Here's the drawing with two shaded views (mm, measured from the low corner). I have some questions. A direction names the side the tool comes from. Give positions to 0.01 mm unless a question says otherwise; leave off trailing zeros. Write each loop counter-clockwise with the first axis right and the second up, starting at its lowest first coordinate (ties: lowest second). Pieces come first, ordered by that corner, then holes.
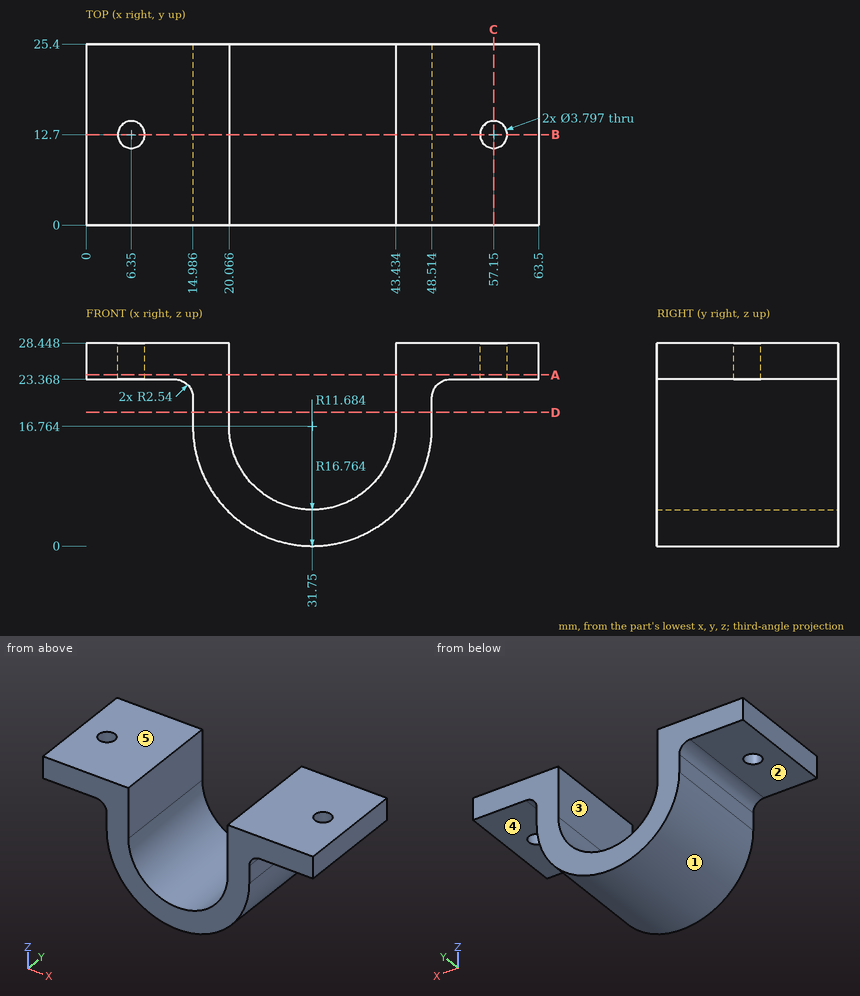
(1) Imagine slicing it at B-B, the plane y = 12.7. Write out the boundary of the cut face in (x, z).
Returned:
outline: (0, 23.37) - (4.45, 23.37) - (4.45, 28.45) - (0, 28.45) - close; (8.25, 23.37) - (12.45, 23.37) arc R2.54 cw to (14.99, 20.83) - (14.99, 16.76) arc R16.76 ccw to (48.51, 16.76) - (48.51, 20.83) arc R2.54 cw to (51.05, 23.37) - (55.25, 23.37) - (55.25, 28.45) - (43.43, 28.45) - (43.43, 16.76) arc R11.68 cw to (20.07, 16.76) - (20.07, 28.45) - (8.25, 28.45) - close; (59.05, 23.37) - (63.5, 23.37) - (63.5, 28.45) - (59.05, 28.45) - close
(2) Will these pins go through, and if not, where does the flat tip stop? P1, Ø3.5, axis at x = 58.5, y = 17.5, coming from the -Z side; P2, Ø8, axis at x = 9, z = 18.5, coming from the -Y side; P3, Ø4.5, axis at y = 19, z = 18.5, coming from the +X side; P4, Ø9.5, axis at y = 17, z = 23.5, coming from the -X side.
Returned:
P1: stops at z = 23.37
P2: passes through
P3: stops at x = 48.51
P4: stops at x = 0
(3) Imagine slicing it at C-C, the plane x = 57.15. Write out the boundary of the cut face in (y, z).
Returned:
outline: (0, 23.37) - (10.8, 23.37) - (10.8, 28.45) - (0, 28.45) - close; (14.6, 23.37) - (25.4, 23.37) - (25.4, 28.45) - (14.6, 28.45) - close
(4) If I drill on L1, parallel to X at y = 12.7, z = 25.75; L2, parallel to Y at x = 6.35, z = 26.8; L3, parallel to X at y = 5.75, z = 20, over which ranges is the centre line in solid material (lowest first)?
Returned:
L1: x = 0 to 4.45, 8.25 to 20.07, 43.43 to 55.25, 59.05 to 63.5
L2: y = 0 to 10.8, 14.6 to 25.4
L3: x = 14.99 to 20.07, 43.43 to 48.51
(5) Imagine slicing it at D-D, the plane z = 18.75. Write out the boundary of the cut face in (x, y).
Returned:
outline: (14.99, 0) - (20.07, 0) - (20.07, 25.4) - (14.99, 25.4) - close; (43.43, 0) - (48.51, 0) - (48.51, 25.4) - (43.43, 25.4) - close
(6) For the marked faces 1, 2, 3, 4 and 5, which set-ups out of +Z, -Z, +X, -X, +Y, -Y let a thin tool reach every point of the face, with its end or its side?
Returned:
face 1: -Z, +Y, -Y
face 2: -Z, -X, +Y, -Y
face 3: +Z, +Y, -Y
face 4: -Z, +X, +Y, -Y
face 5: +Z, +X, -X, +Y, -Y
(7) Imagine slicing it at A-A, the plane z = 24. Write out the boundary of the cut face in (x, y).
Returned:
outline: (0, 0) - (20.07, 0) - (20.07, 25.4) - (0, 25.4) - close; (43.43, 0) - (63.5, 0) - (63.5, 25.4) - (43.43, 25.4) - close; hole circle Ø3.8 at (6.35, 12.7); hole circle Ø3.8 at (57.15, 12.7)
